Could you check a few things on this model? Use its own coordinates, in mm. A direction names the side the tool comes from. Give positions to 0.01 mm unless a question says otherwise; leave off trailing zeros. Loops run counter-clockwise (first coordinate to the right, second up) from the corner with the lowest first, then second, coordinate; pieces in that order, holes last. Notation, with made-up numbers: M 33.5,-33.5 L 54.5,-33.5 A13 ccw 54.5,-28.5 Z; hole C 38,-20 d2. An arc over 180 degrees is marked long. Return JSON: item names as keys, results as strings. Group by question number.
1. If we section it at B-B (z = 11): Write out the boundary of the cut face in (x, y) (3 decimals), plus the area to 3 significant figures.
2. If we section it at A-A (x = 0): Write out the boundary of the cut face in (y, z) (3 decimals).
3. For pin 1 (2.5 mm diameter, centred on x = 0, z = 11, fed in from -Y); pin 2 (3 mm diameter, centred on x = 9.5, z = 30.5, fed in from +Y); pin 3 (2 mm diameter, centred on y = -9.5, z = 11.5, fed in from +X); pin 4 (2 mm diameter, centred on y = -4, z = 6, fed in from +X), each with a flat end and sliding along its axis, tell me the tip position at first contact or that it passes through.
4. If we section it at C-C (y = 10.5): Write out the boundary of the cut face in (x, z) (3 decimals).
5. If we section it at D-D (x = 10): Write out the boundary of the cut face in (y, z), plus the area to 3 significant figures.
6. If we mould it in two halves opening along X, with no side actions, what happens to faces 1 (the flat face through (8, 5, 18)), 2 (the flat face through (0, -2.1, 14)), 3 (the flat face through (0, 2.1, 14)), 4 (the flat face through (4.48, 9.93, 7.58))? For each: +X half, -X half, draft (parallel to the pull), parting line (faces both ways), or undercut.
7. Please list where these lines run through material, in increasing order: line 1 (Z direction, x = 0, y = -7.5) (3 decimals); line 2 (Y direction, x = 1.5, z = 32); line 3 (Y direction, x = -3, z = 9.5).
8. For faces 5 (the flat face through (-5.037, 9.93, 19.938)), 6 (the flat face through (5.064, 9.93, 19.812)), 7 (the flat face through (11.72, -0.03, 17.26)), which set-ups out of +Z, -Z, +X, -X, +Y, -Y let a thin tool reach every point of the face, with its end or its side?
```python
from build123d import *

# Parameters (mm, degrees)
F1_DEPTH = 5
F3_DEPTH = 2.1
F4_R     = 1.375
F4_R_2   = 2
F5_DEPTH = 15
F6_W     = 3.8688962813
F6_H     = 4.2
F6_W_2   = 6.0080378316
F6_W_3   = 3.8534507621
F7_DEPTH = 35.001
F8_DEPTH = 20.001


with BuildPart() as f1:
    # F0 (on Front) → F1 (new body, symmetric)
    with BuildSketch(Plane.XZ):
        Polygon((-10.5, 35), (-19, 0), (19, 0), (10.5, 35), align=None)
    extrude(amount=F1_DEPTH, both=True)

    # F2 (on Front) → F3 (cut, symmetric)
    with BuildSketch(Plane.XZ):
        Polygon((-7.4127979777, 35), (-16.0847388882, -0.7079919843), (16.0847388882, -0.7079919843), (7.4127979777, 35), align=None)
    extrude(amount=F3_DEPTH, both=True, mode=Mode.SUBTRACT)

    # F4 (on Front) → F5 (join, symmetric)
    with BuildSketch(Plane.XZ):
        Polygon((4.1015339084, 24.375), (-4.1015339084, 24.375), (-6, 15.375), (-3.0040189158, 0), (3.0040189158, 0), (6, 15.375), align=None)
        with Locations((0, 11)):
            Circle(F4_R, mode=Mode.SUBTRACT)
        with Locations((0, 17.375)):
            Circle(F4_R_2, mode=Mode.SUBTRACT)
    extrude(amount=F5_DEPTH, both=True)

    # F6 (on face) → F7 (cut, through all)
    with BuildSketch(Plane(origin=(0, 0, 0), x_dir=(1, 0, 0), z_dir=(0, 0, -1))):
        with Locations((-4.9384670565, 0)):
            Rectangle(F6_W, F6_H)
        Rectangle(F6_W_2, F6_H)
        with Locations((4.9307442969, 0)):
            Rectangle(F6_W_3, F6_H)
    extrude(amount=-F7_DEPTH, mode=Mode.SUBTRACT)

    # F8 (cut, through all): faces of the model
    f8_faces = [f1.faces().sort_by_distance(p)[0] for p in [
        (0, 5, 17.375),
        (0, 5, 11),
    ]]
    extrude(f8_faces, amount=-F8_DEPTH, mode=Mode.SUBTRACT)


solid = f1.part
```
Answer:
{
 "1": {"outline": "M -16.329,-5 L -5.147,-5 L -5.147,-15 L -1.375,-15 L -1.375,-2.1 L -13.241,-2.1 L -13.241,2.1 L -1.375,2.1 L -1.375,15 L -5.147,15 L -5.147,5 L -16.329,5 Z; M 1.375,-15 L 5.147,-15 L 5.147,-5 L 16.329,-5 L 16.329,5 L 5.147,5 L 5.147,15 L 1.375,15 L 1.375,2.1 L 13.241,2.1 L 13.241,-2.1 L 1.375,-2.1 Z", "area": "350 mm²"},
 "2": {"outline": "M -15,0 L -2.1,0 L -2.1,9.625 L -15,9.625 Z; M -15,12.375 L -2.1,12.375 L -2.1,15.375 L -15,15.375 Z; M -15,19.375 L -2.1,19.375 L -2.1,35 L -5,35 L -5,24.375 L -15,24.375 Z; M 2.1,0 L 15,0 L 15,9.625 L 2.1,9.625 Z; M 2.1,12.375 L 15,12.375 L 15,15.375 L 2.1,15.375 Z; M 2.1,19.375 L 15,19.375 L 15,24.375 L 5,24.375 L 5,35 L 2.1,35 Z"},
 "3": {"pin 1": "passes through", "pin 2": "stops at y = 5", "pin 3": "stops at x = 5.44", "pin 4": "stops at x = 17.79"},
 "4": {"outline": "M -6,15.375 L -3.004,0 L 3.004,0 L 6,15.375 L 4.102,24.375 L -4.102,24.375 Z; hole C 0,17.375 d4; hole C 0,11 d2.75"},
 "5": {"outline": "M -5,0 L -2.1,0 L -2.1,24.35 L 2.1,24.35 L 2.1,0 L 5,0 L 5,35 L -5,35 Z", "area": "248 mm²"},
 "6": {"face 1": "draft", "face 2": "undercut", "face 3": "undercut", "face 4": "+X half"},
 "7": {"line 1": "z = 0 to 9.625, 12.375 to 15.375, 19.375 to 24.375", "line 2": "y = -5 to -2.1, 2.1 to 5", "line 3": "y = -15 to -2.1, 2.1 to 15"},
 "8": {"face 5": "+Z, -X, +Y", "face 6": "+Z, +X, +Y", "face 7": "-Z"}
}
